Part model, mm, in its own coordinate system. Face numbers are marked on the shaded views. A direction names the side the tool comes from. Coordinates: 2 decimals unless noted, no trailing zeros. Write each loop counter-clockwise with the first axis right and the second up, starting at its lowest first coordinate (ties: lowest second). Pieces come first, ordered by that corner, then holes. Notation, with made-up numbers: M 74.25,72 L 122.25,72 A24 cw 122.25,83 Z; hole C 18.5,-29 d3. An arc over 180 degrees is marked long. Use a Markdown table: item, result. Add a question column.
Q1. Slice it at C-C on z = 0.85. Write the cut outline in (x, y), then the cut area to 3 significant figures.
Q2. Slice it at A-A on z = 4.35. Write the cut outline in (x, y) (1 decimal).
Q3. Pin check, flat tip, straight feed: pin 1 Ø3 at (x, z) = (3.5, 4) entering from +Y. Stop position of the tip, or through.
Q4. Mould opens along X. For the marked faces 1, 2, 3 and 4 say: released by +X, released by -X, zero draft, split by the parting line, or undercut.
Q5. Tool access for the marked faces 5, 6 and 7: list every direction of +Z, -Z, +X, -X, +Y, -Y with a clear straight run to the whole face (end or side of a thin tool).
Q6. Wall check: L1, parallel to X at y = 1.25, z = 1.4; L2, parallel to X at y = 0.5, z = 0.7; L3, parallel to Y at x = -1, z = 0.5. Give the ranges that are in metal, low to high. Write a range as from..to.
Autodesk Inventor part; units mm, degrees
ref_plane "YZ Plane" through (0, 0, 0) normal (1, 0, 0) x (0, 1, 0)
ref_plane "XZ Plane" through (0, 0, 0) normal (0, 1, 0) x (-1, 0, 0)
ref_plane "XY Plane" through (0, 0, 0) normal (0, 0, 1) x (1, 0, 0)
sketch "Sketch1" plane through (0, 0, 0) normal (0, 0, 1) x (1, 0, 0)
  circle A0 centre (0, 0) radius 4.5085
  dimension "d0" = 9.017
extrude "Extrusion1" add sketch "Sketch1" along normal blind 5.08
sketch "Sketch2" plane through (0, 0, 0) normal (0, 0, -1) x (-1, 0, 0)
  circle A0 centre (0, 0) radius 3.81
  dimension "d3" = 7.62
extrude "Extrusion2" add sketch "Sketch2" along normal blind 0.635 draft -15
sketch "Sketch3" plane through (0, 0, 5.08) normal (0, 0, 1) x (1, 0, 0)
  circle A0 centre (0, 0) radius 4.1275
  circle A1 centre (0, 0) radius 4.5085
  dimension "d6" = 8.255
extrude "Extrusion3" cut sketch "Sketch3" against normal blind 1.27
chamfer "Chamfer1" distance 0.381 angle 45 1 edges at (-4.1275, 0, 5.08)
sketch "Sketch4" plane through (0, 0, 5.08) normal (0, 0, 1) x (1, 0, 0)
  circle A0 centre (0, 0) radius 2.3813 construction
  line L0 (-2.3813, 1.3748) -> (0, 2.7496)
  line L1 (0, 2.7496) -> (2.3812, 1.3748)
  line L2 (2.3812, 1.3748) -> (2.3813, -1.3748)
  line L3 (2.3813, -1.3748) -> (0, -2.7496)
  line L4 (0, -2.7496) -> (-2.3812, -1.3748)
  line L5 (-2.3812, -1.3748) -> (-2.3813, 1.3748)
  point P0 (-2.3813, 0)
  dimension "d12" = 4.7625
extrude "Extrusion4" cut sketch "Sketch4" against normal through all
thread "Thread1"
properties part number "Pillow Ball Retainer"
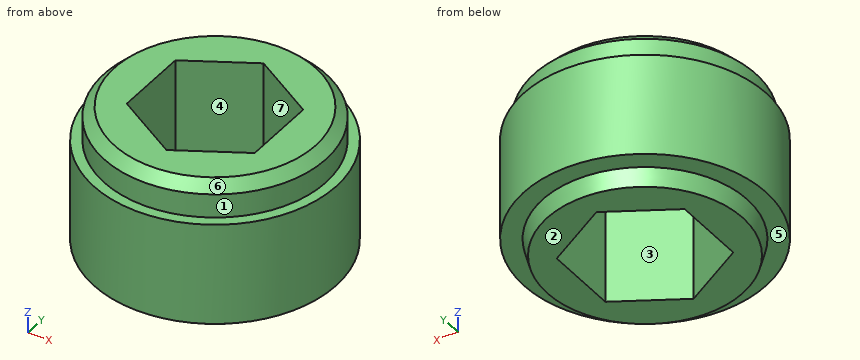
Recorded:
| question | item | result |
|---|---|---|
| 1 | outline | C 0,0 d9.02; hole M -2.38,-1.37 L 0,-2.75 L 2.38,-1.37 L 2.38,1.37 L 0,2.75 L -2.38,1.37 Z |
| 1 | area | 44.2 mm² |
| 2 | outline | C 0,0 d8.3; hole M -2.4,-1.4 L 0,-2.7 L 2.4,-1.4 L 2.4,1.4 L 0,2.7 L -2.4,1.4 Z |
| 3 | pin 1 | y = 4.03 |
| 4 | face 1 | split by the parting line |
| 4 | face 2 | zero draft |
| 4 | face 3 | undercut |
| 4 | face 4 | undercut |
| 5 | face 5 | -Z |
| 5 | face 6 | +Z |
| 5 | face 7 | +Z, -Z |
| 6 | L1 | -4.33..-2.38, 2.38..4.33 |
| 6 | L2 | -4.48..-2.38, 2.38..4.48 |
| 6 | L3 | -4.4..-2.17, 2.17..4.4 |
